```python
from build123d import *

# Parameters (mm, degrees)
SKETCH_2_W          = 7
SKETCH_2_H          = 7
CUT_EXTRUDE_1_DEPTH = 32.8


with BuildPart() as part:
    # Эскиз1 → Повернуть1 (revolve)
    with BuildSketch(Plane(origin=(0, 0, 0), x_dir=(0, 0, -1), z_dir=(1, 0, 0))):
        Polygon((26.8, 12.5), (-5, 12.5), (-5, 16.5), (1.5, 16.5), (1.5, 18), (23, 18), (23, 19.5), (26.8, 19.5), align=None)
    revolve(axis=Axis((0, 0, 1000), (0, 0, -1)))

    # Эскиз2 → Вырез-Вытянуть1 (cut, through all)
    with BuildSketch(Plane.XY.offset(5)):
        with Locations((0, 12.5)):
            Rectangle(SKETCH_2_W, SKETCH_2_H)
    extrude(amount=-CUT_EXTRUDE_1_DEPTH, mode=Mode.SUBTRACT)


solid = part.part
```
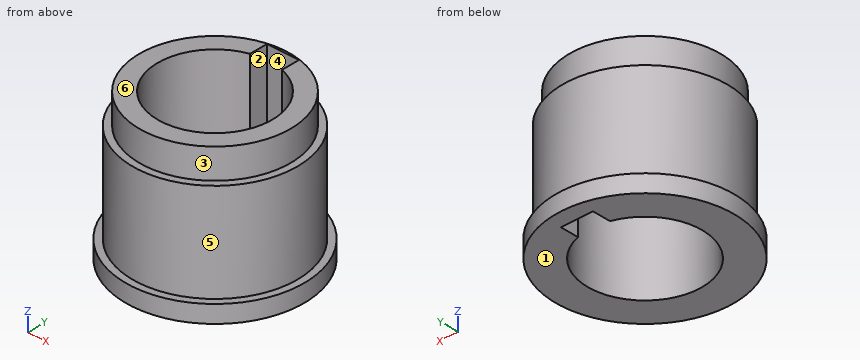
The listing builds one solid part. Answer for the finished solid, in the listing's coordinates (mm). Face numbers are marked on the shaded views. A direction names the side the tool comes from. Round coordinates to 2 decimals unless told otherwise and drop trailing zeros. Loops run counter-clockwise (first coordinate to the right, second up) from the corner with the lowest first, then second, coordinate; pieces in that order, holes last.
Q1. Find the intervals of material crossed by line 1 (X direction, y = 0, z = -14); line 2 (Y direction, x = -8, z = -17.5); line 3 (X direction, y = -6, z = -24.5), in increasing order.
Q2. Section A-A, the plane y = 0 is taken. Determine the outline of the cut face in (x, z).
Q3. Given pin 1 Ø6 at (x, z) = (-14.5, 1) entering from -Y; pin 2 Ø1.5 at (y, z) = (-2, -23) entering from -X; pin 3 Ø2 at (x, z) = (-12, -7.5) entering from +Y, each flat-ended and moving along its own axis, determine where each tip first touches the part or whether it passes through.
Q4. Section D-D, the plane z = -0.5 is taken. Determine the outline of the cut face in (x, y).
Q5. Section C-C, the plane z = -12 is taken. Determine the outline of the cut face in (x, y).
Q6. Section B-B, the plane x = 0 is taken. Determine the outline of the cut face in (y, z), then the cut area to 3 significant figures.
Q7. Which of the six approach directions +Z, -Z, +X, -X, +Y, -Y give full straight-line access (tool end or side, diameter ignored) to the marked faces 1, 2 and 3?
Q8. For a pull along X with two mould halves and no side action, classify the marked faces 4, 5 and 6 as released by +X, released by -X, zero draft, split by the parting line, or undercut.
Completed:
1. line 1: x = -18 to -12.5, 12.5 to 18
1. line 2: y = -16.12 to -9.6, 9.6 to 16.12
1. line 3: x = -18.55 to -10.97, 10.97 to 18.55
2. outline: (-19.5, -26.8) - (-12.5, -26.8) - (-12.5, 5) - (-16.5, 5) - (-16.5, -1.5) - (-18, -1.5) - (-18, -23) - (-19.5, -23) - close; (12.5, -26.8) - (19.5, -26.8) - (19.5, -23) - (18, -23) - (18, -1.5) - (16.5, -1.5) - (16.5, 5) - (12.5, 5) - close
3. pin 1: stops at y = -12.61
3. pin 2: stops at x = -19.46
3. pin 3: stops at y = 14.25
4. outline: circle Ø33 at (0, 0); hole (-3.5, 12) arc R12.5 ccw (long way) to (3.5, 12) - (3.5, 16) - (-3.5, 16) - close
5. outline: circle Ø36 at (0, 0); hole (-3.5, 12) arc R12.5 ccw (long way) to (3.5, 12) - (3.5, 16) - (-3.5, 16) - close
6. outline: (-19.5, -26.8) - (-12.5, -26.8) - (-12.5, 5) - (-16.5, 5) - (-16.5, -1.5) - (-18, -1.5) - (-18, -23) - (-19.5, -23) - close; (16, -26.8) - (19.5, -26.8) - (19.5, -23) - (18, -23) - (18, -1.5) - (16.5, -1.5) - (16.5, 5) - (16, 5) - close
6. area: 230 mm2
7. face 1: -Z, +X, -X, +Y, -Y
7. face 2: +Z, -Z
7. face 3: +Z
8. face 4: undercut
8. face 5: split by the parting line
8. face 6: zero draft
